from build123d import *

# Parameters (mm, degrees)
BOSS_EXTRU_1_DEPTH      = 32
ESQUISSE2_R             = 4
ENL_V_MAT_EXTRU_1_DEPTH = 32
ESQUISSE3_R             = 4.5
ENL_V_MAT_EXTRU_3_DEPTH = 42
ENL_V_MAT_EXTRU_4_DEPTH = 8.5
BOSS_EXTRU_2_DEPTH      = 20
ESQUISSE7_R             = 12
ENL_V_MAT_EXTRU_5_DEPTH = 33


with BuildPart() as part:
    # Esquisse1 → Boss.-Extru.1 (new body)
    with BuildSketch(Plane.XY):
        with BuildLine():
            Line((-27.461265237, 12.171141476), (28.529805479, 12.171141476))
            ThreePointArc((28.529805479, 12.171141476), (32.534270121, -3.328858524), (28.529805479, -18.828858524))
            Line((28.529805479, -18.828858524), (-27.461265237, -18.828858524))
            ThreePointArc((-27.461265237, -18.828858524), (-31.465729879, -3.328858524), (-27.461265237, 12.171141476))
        make_face()
    extrude(amount=BOSS_EXTRU_1_DEPTH)

    # Esquisse2 → Enlèv. mat.-Extru.1 (cut)
    with BuildSketch(Plane.XZ.offset(18.828858524)):
        with Locations(Location((24.534270121, 21, 0), (0, 0, 357.292669089))):
            Circle(ESQUISSE2_R)
        with Locations(Location((-23.465729879, 21, 0), (0, 0, 182.707330911))):
            Circle(ESQUISSE2_R)
    extrude(amount=-ENL_V_MAT_EXTRU_1_DEPTH, mode=Mode.SUBTRACT)

    # Esquisse3 → Enlèv. mat.-Extru.3 (cut)
    with BuildSketch(Plane.XY):
        with Locations((-24, 4.671141476)):
            Circle(ESQUISSE3_R)
        with Locations(Location((24, 4.671141476, 0), (0, 0, 180))):
            Circle(ESQUISSE3_R)
    extrude(amount=ENL_V_MAT_EXTRU_3_DEPTH, mode=Mode.SUBTRACT)

    # Esquisse5 → Enlèv. mat.-Extru.4 (cut)
    with BuildSketch(Plane.XZ.offset(18.828858524)):
        with BuildLine():
            Line((-15.465729879, 32), (-15.465729879, 24))
            ThreePointArc((-15.465729879, 24), (-17.80887563, 18.343145751), (-23.465729879, 16))
            Line((-23.465729879, 16), (-31.465729879, 16))
            Line((-31.465729879, 16), (-31.465729879, 32))
            Line((-31.465729879, 32), (-15.465729879, 32))
        make_face()
        with BuildLine():
            Line((24.534270121, 16), (32.534270121, 16))
            Line((32.534270121, 16), (32.534270121, 32))
            Line((32.534270121, 32), (16.534270121, 32))
            Line((16.534270121, 32), (16.534270121, 24))
            ThreePointArc((16.534270121, 24), (18.877415871, 18.343145751), (24.534270121, 16))
        make_face()
    extrude(amount=-ENL_V_MAT_EXTRU_4_DEPTH, mode=Mode.SUBTRACT)

    # Esquisse6 → Boss.-Extru.2 (add)
    with BuildSketch(Plane.XY.offset(32)):
        with BuildLine():
            Line((9.643650761, 12.171141476), (-9.643650761, 12.171141476))
            ThreePointArc((-9.643650761, 12.171141476), (-7.907526069, -16.877813022), (17, -1.828858524))
            ThreePointArc((17, -1.828858524), (15.048954498, 6.078667545), (9.643650761, 12.171141476))
        make_face()
    extrude(amount=BOSS_EXTRU_2_DEPTH)

    # Esquisse7 → Enlèv. mat.-Extru.5 (cut)
    with BuildSketch(Plane.XY.offset(52)):
        with Locations((0.177122326, -1.910835069)):
            Circle(ESQUISSE7_R)
    extrude(amount=-ENL_V_MAT_EXTRU_5_DEPTH, mode=Mode.SUBTRACT)


solid = part.part
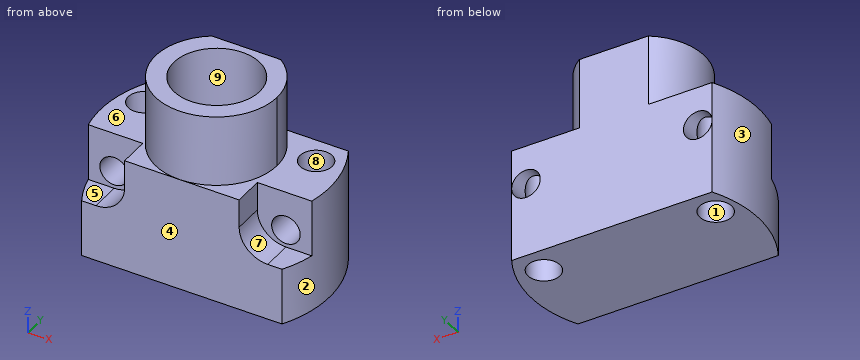
CAD build for the part. Positions are in the model's coordinates, mm. Face numbers are marked on the shaded views. A direction names the side the tool comes from. Give positions to 0.01 mm unless a question says otherwise; leave off trailing zeros. Loops run counter-clockwise (first coordinate to the right, second up) from the corner with the lowest first, then second, coordinate; pieces in that order, holes last. Notation, with made-up numbers: M -6.5,38 L 46.5,38 A21 cw 46.5,59 Z; hole C 27.5,31.25 d9. An arc over 180 degrees is marked long. Answer in a Markdown table with one row per item. Add a question column.
Item 1: Drop flat-ended pins along their axis: P1, Ø9, axis at y = -14, z = 28, coming from the -X side; P2, Ø2.5, axis at y = -15.5, z = 28.5, coming from the +X side; P3, Ø6, axis at x = -27, y = -14.5, coming from the +Z side; P4, Ø8, axis at x = 24, y = 4.67, coming from the -Z side. Give the stop position or say it passes through.
Item 2: Mould opens along X. For the marked faces 1, 2, 3 and 4 say: +X half, -X half, draft (parallel to the pull), parting line (faces both ways), or undercut.
Item 3: Band-saw the part on C-C on x = 2.5. Give the cut face in (y, z), then the cut area to 3 significant figures.
Item 4: Probe probe 1 along X at (y, z) = (-1, 21); probe 2 along X at (y, z) = (2, 17.5); probe 3 along X at (y, z) = (6, 29.5). List the from-to ranges inside material, lowest first.
Item 5: Band-saw the part on D-D on z = 30. Give the cut face in (x, y), then the cut area to 3 significant figures.
Item 6: Band-saw the part on A-A on y = -5. Give the cut face in (x, z).
Item 7: Band-saw the part on B-B on z = 14.5. Give the cut face in (x, y).
Item 8: Tool access for the marked faces 5, 6, 7, 8 and 9: list every direction of +Z, -Z, +X, -X, +Y, -Y with a clear straight run to the whole face (end or side of a thin tool).
Reply:
| question | item | result |
|---|---|---|
| 1 | P1 | stops at x = -30.87 |
| 1 | P2 | stops at x = 16.53 |
| 1 | P3 | stops at z = 16 |
| 1 | P4 | passes through |
| 2 | face 1 | undercut |
| 2 | face 2 | +X half |
| 2 | face 3 | -X half |
| 2 | face 4 | draft |
| 3 | outline | M -18.83,0 L 12.17,0 L 12.17,52 L 9.86,52 L 9.86,19 L -13.68,19 L -13.68,52 L -18.64,52 L -18.64,32 L -18.83,32 Z |
| 3 | area | 831 mm^2 |
| 4 | probe 1 | x = -31.38 to -27.47, -19.47 to -11.79, 12.14 to 20.53, 28.53 to 32.45 |
| 4 | probe 2 | x = -31.02 to -27.62, -20.38 to 20.38, 27.62 to 32.09 |
| 4 | probe 3 | x = -30.08 to -28.3, -19.7 to -8.85, 9.2 to 19.7, 28.3 to 31.14 |
| 5 | outline | M -30.69,-10.33 L -15.47,-10.33 L -15.47,-18.83 L 16.53,-18.83 L 16.53,-10.33 L 31.76,-10.33 A32 ccw 28.53,12.17 L -27.46,12.17 A32 ccw Z; hole C -24,4.67 d9; hole C 0.18,-1.91 d24; hole C 24,4.67 d9 |
| 5 | area | 1,090 mm^2 |
| 6 | outline | M -31.42,0 L 32.49,0 L 32.49,32 L 16.7,32 L 16.7,52 L 11.77,52 L 11.77,19 L -11.42,19 L -11.42,52 L -16.7,52 L -16.7,32 L -31.42,32 Z; hole C -23.47,21 d8; hole C 24.53,21 d8 |
| 7 | outline | M -27.46,-18.83 L 28.53,-18.83 A32 ccw 28.53,12.17 L -27.46,12.17 A32 ccw Z; hole C -24,4.67 d9; hole C 24,4.67 d9 |
| 8 | face 5 | +Z, -X, -Y |
| 8 | face 6 | +Z, -X |
| 8 | face 7 | +Z, +X, -Y |
| 8 | face 8 | +Z, -Z |
| 8 | face 9 | +Z |
